The figure shows three views and two pictorial views of one solid part (mm, origin at its lowest corner). Answer the questions. Coordinates: 2 decimals unless noted, no trailing zeros.
Item 1: Straight lines are drawn through the part: probe 1 along Z at (x, y) = (12.5, 6) (1 decimal); probe 2 along X at (y, z) = (6.5, 13) (1 decimal); probe 3 along X at (y, z) = (4.75, 58.5) (1 decimal). For each, find the intervals that lie inside material, in ascending order.
Item 2: Section A-A (y = 3.75) is taken. State how many separate pieces and enclosed holes the cut face has, then the cut area to 3 significant figures.
Item 3: This flat-tipped pin is pushed along its axis until it touches: P1, Ø3, axis at x = 14, z = 61, coming from the -Y side. Where does it stop, or does it pass through?
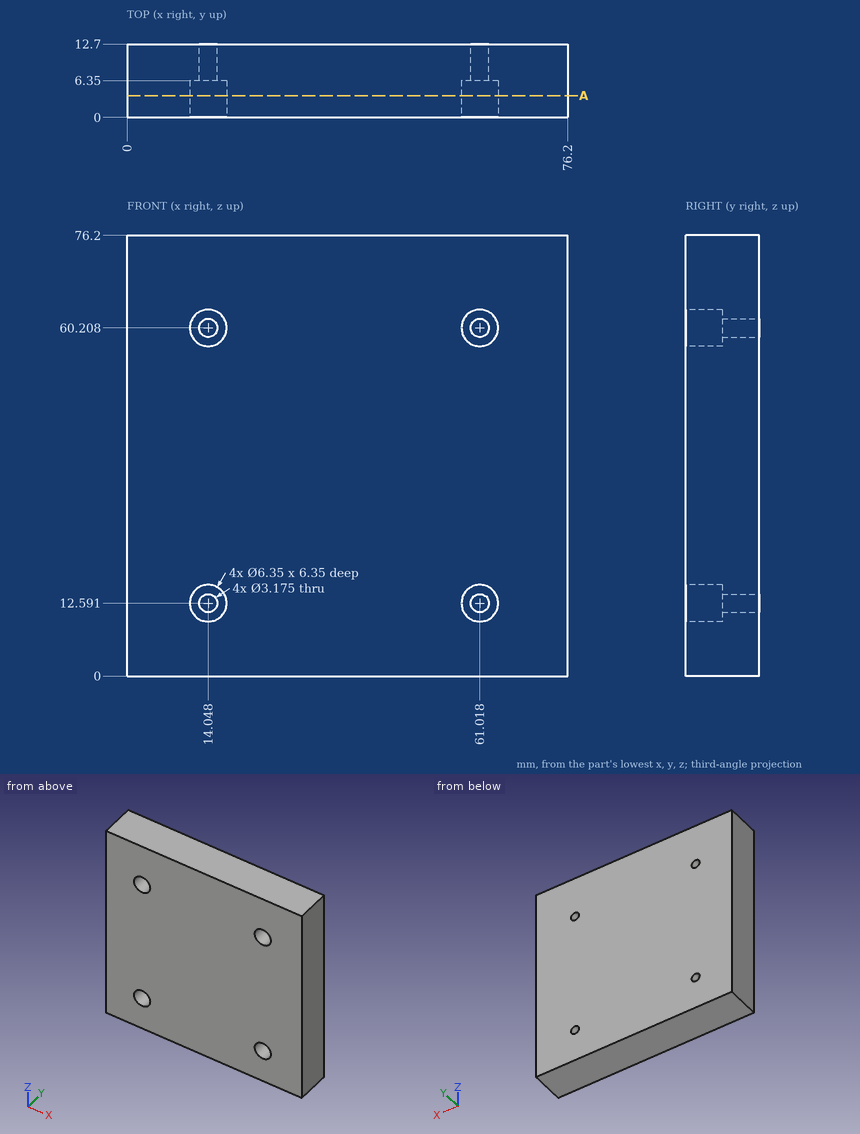
Established:
1. probe 1: z = 0 to 9.8, 15.4 to 57.4, 63 to 76.2
1. probe 2: x = 0 to 12.5, 15.6 to 59.5, 62.6 to 76.2
1. probe 3: x = 0 to 11.4, 16.7 to 58.3, 63.7 to 76.2
2. separate pieces: 1
2. enclosed holes: 4
2. area: 5,680 mm2
3. P1: stops at y = 6.35
